```python
from build123d import *

# Parameters (mm, degrees)
BASPROSKE_W     = 5
BASPROSKE_H     = 7
TOOTHCUT_DEPTH  = 12.090536506
TEETHCUTS_COUNT = 12
TEETHCUTS_ANGLE = 330
BORSKE_R        = 2.5
BORE_DEPTH      = 50.0000508
REDONDEO1_R     = 2


with BuildPart() as part:
    # BasProSke → Base-Revolve (revolve)
    with BuildSketch(Plane(origin=(0, 0, 0), x_dir=(1, 0, 0), z_dir=(0, 1, 0)), mode=Mode.PRIVATE) as base_revolve_sk:
        with Locations((2.5, 3.5)):
            Rectangle(BASPROSKE_W, BASPROSKE_H)
    revolve(base_revolve_sk.sketch.rotate(Axis((-10, 0, 0), (1, 0, 0)), 180), axis=Axis((-10, 0, 0), (1, 0, 0)))

    # TooCutSke → ToothCut (cut, through all)
    with BuildSketch(Plane(origin=(0, 0, 0), x_dir=(0, 0, -1), z_dir=(1, 0, 0))):
        with BuildLine():
            ThreePointArc((0.562207301, 4.715604304), (0, 4.749), (-0.562207301, 4.715604304))
            ThreePointArc((-0.562207301, 4.715604304), (-0.837528627, 5.917009812), (-1.672850686, 6.823328788))
            ThreePointArc((-1.672850686, 6.823328788), (0, 7.0254), (1.672850686, 6.823328788))
            ThreePointArc((1.672850686, 6.823328788), (0.837528627, 5.917009812), (0.562207301, 4.715604304))
        make_face()
    toothcut = extrude(amount=TOOTHCUT_DEPTH, mode=Mode.SUBTRACT)

    # TeethCuts: ToothCut ×12 about axis
    teethcuts_axis = Axis((-10, 0, 0), (1, 0, 0))
    for i in range(1, TEETHCUTS_COUNT):
        add(toothcut.rotate(teethcuts_axis, i * TEETHCUTS_ANGLE / (TEETHCUTS_COUNT - 1)), mode=Mode.SUBTRACT)

    # BorSke → Bore (cut, symmetric)
    with BuildSketch(Plane(origin=(0, 0, 0), x_dir=(0, 0, -1), z_dir=(1, 0, 0))):
        with Locations(Location((0, 0, 0), (0, 0, 180))):
            Circle(BORSKE_R)
    extrude(amount=BORE_DEPTH, both=True, mode=Mode.SUBTRACT)

    # Redondeo1
    redondeo1_edges = [part.edges().sort_by_distance(p)[0] for p in [
        (5, 0, -2.5),
    ]]
    fillet(redondeo1_edges, radius=REDONDEO1_R)


solid = part.part
```
For this review, take the finished solid that the model builds, in its own axes (mm). Coordinates: 2 decimals unless noted, no trailing zeros. Loops run counter-clockwise (first coordinate to the right, second up) from the corner with the lowest first, then second, coordinate; pieces in that order, holes last.
1. Mouldability with a two-part tool opening along Y and no side actions: class faces 1 (the cylindrical face through (1.5, -0.1, -2.5)), 2 (the cylindrical face through (2.5, -4.1, -2.4)) as +Y half, -Y half, draft (parallel to the pull), parting line (faces both ways), or undercut.
2. For line 1 (Y direction, x = 0.4, z = 4.5); line 2 (Z direction, x = 0.45, y = -4); line 3 (Y direction, x = 0.25, z = 5.25), list the stretches that pass through material, from the lowest coordinate up.
3. Add section A-A, the plane y = 0. Give the boundary of the cut face in (x, z).
4. Insertion check: P1, Ø1, axis at x = 3, z = 1, coming from the +Y side; P2, Ø1, axis at x = 1, y = -5, coming from the +Z side. Each pin has a flat end and moves straight along its axis. Give the tip position at first contact, or say it passes through.
Result:
1. face 1: undercut
1. face 2: undercut
2. line 1: y = -5.03 to -3.4, -1.95 to 1.95, 3.4 to 5.03
2. line 2: z = -4.87 to -2.96, -2.56 to 2.56, 2.96 to 4.87
2. line 3: y = -2.2 to -0.6, 0.6 to 2.2
3. outline: (0, -4.75) - (5, -4.75) - (5, -4.5) arc R2 ccw to (3, -2.5) - (0, -2.5) - close; (0, 2.5) - (3, 2.5) arc R2 ccw to (5, 4.5) - (5, 4.75) - (0, 4.75) - close
4. P1: stops at y = 6.7
4. P2: stops at z = 5.07
